Here's how the part is built. I have some questions about the finished solid (model axes, mm). Coordinates: 2 decimals unless noted, no trailing zeros. Write each loop counter-clockwise with the first axis right and the second up, starting at its lowest first coordinate (ties: lowest second). Pieces come first, ordered by that corner, then holes. Notation, with made-up numbers: M 82.5,-25.75 L 106.5,-25.75 A10 cw 106.5,-10.75 Z; hole C -30,16.5 d1. An arc over 180 degrees is marked long. Use a Markdown table: item, result.
```python
from build123d import *

# Parameters (mm, degrees)
SKETCH2_W                      = 53.34
SKETCH2_H                      = 17.780149528
BOSS_EXTRUDE1_DEPTH            = 1.524
F_2_CLEARANCE_HOLE1_AT_2_COUNT = 2
F_2_CLEARANCE_HOLE1_AT_2_PITCH = 13.038661485
F_2_CLEARANCE_HOLE1_AT_3_COUNT = 2
F_2_CLEARANCE_HOLE1_AT_3_PITCH = 50.333486658
F_2_CLEARANCE_HOLE1_AT_4_COUNT = 2
F_2_CLEARANCE_HOLE1_AT_4_PITCH = 48.615359567
FILLET1_R                      = 1.27
CUT_EXTRUDE1_REACH             = 30.154
SKETCH6_R                      = 6.35
FILLET2_R                      = 0.254


with BuildPart() as part:
    # Sketch2 → Boss-Extrude1 (new body)
    with BuildSketch(Plane.XY):
        Rectangle(SKETCH2_W, SKETCH2_H)
    extrude(amount=-BOSS_EXTRUDE1_DEPTH)

    # Sketch4 → #2 Clearance Hole1 (revolve, cut)
    with BuildSketch(Plane(origin=(-24.307679783, 6.519330742, 0), x_dir=(0, -1, 0), z_dir=(1, 0, 0))):
        Polygon((0, 0), (0, 1.524), (1.2192, 1.524), (1.2192, 0.635), (1.8542, 0), align=None)
    f_2_clearance_hole1 = revolve(axis=Axis((-24.307679783, 6.519330742, 6.35), (0, 0, -1)), mode=Mode.SUBTRACT)

    # #2 Clearance Hole1 at 2: #2 Clearance Hole1 ×2
    with Locations(*[(0, -i * F_2_CLEARANCE_HOLE1_AT_2_PITCH, 0) for i in range(1, F_2_CLEARANCE_HOLE1_AT_2_COUNT)]):
        add(f_2_clearance_hole1, mode=Mode.SUBTRACT)

    # #2 Clearance Hole1 at 3: #2 Clearance Hole1 ×2
    with Locations(*[Vector(0.9658651286657962, -0.25904546556040114, 0) * (i * F_2_CLEARANCE_HOLE1_AT_3_PITCH) for i in range(1, F_2_CLEARANCE_HOLE1_AT_3_COUNT)]):
        add(f_2_clearance_hole1, mode=Mode.SUBTRACT)

    # #2 Clearance Hole1 at 4: #2 Clearance Hole1 ×2
    with Locations(*[(i * F_2_CLEARANCE_HOLE1_AT_4_PITCH, 0, 0) for i in range(1, F_2_CLEARANCE_HOLE1_AT_4_COUNT)]):
        add(f_2_clearance_hole1, mode=Mode.SUBTRACT)

    # Fillet1
    fillet1_edges = [part.edges().sort_by_distance(p)[0] for p in [
        (-26.67, 8.890074764, -0.762),
        (26.67, 8.890074764, -0.762),
        (26.67, -8.890074764, -0.762),
        (-26.67, -8.890074764, -0.762),
    ]]
    fillet(fillet1_edges, radius=FILLET1_R)

    # Sketch6 → Cut-Extrude1 (cut, up to next)
    with BuildSketch(Plane.XY, mode=Mode.PRIVATE) as cut_extrude1_sk1:
        Circle(SKETCH6_R)
    cut_extrude1_tool1 = extrude(cut_extrude1_sk1.sketch, amount=-CUT_EXTRUDE1_REACH, mode=Mode.PRIVATE) & part.part
    # Sketch6 → Cut-Extrude1 (cut, up to next)
    with BuildSketch(Plane.XY, mode=Mode.PRIVATE) as cut_extrude1_sk2:
        with Locations((-17.78, 0)):
            Circle(SKETCH6_R)
    cut_extrude1_tool2 = extrude(cut_extrude1_sk2.sketch, amount=-CUT_EXTRUDE1_REACH, mode=Mode.PRIVATE) & part.part
    # Sketch6 → Cut-Extrude1 (cut, up to next)
    with BuildSketch(Plane.XY, mode=Mode.PRIVATE) as cut_extrude1_sk3:
        with Locations((17.779999999, -0.00017224)):
            Circle(SKETCH6_R)
    cut_extrude1_tool3 = extrude(cut_extrude1_sk3.sketch, amount=-CUT_EXTRUDE1_REACH, mode=Mode.PRIVATE) & part.part
    add(cut_extrude1_tool1.solids().sort_by_distance((0, 0, 0))[0], mode=Mode.SUBTRACT)
    add(cut_extrude1_tool2.solids().sort_by_distance((-17.78, 0, 0))[0], mode=Mode.SUBTRACT)
    add(cut_extrude1_tool3.solids().sort_by_distance((17.78, -0.000172, 0))[0], mode=Mode.SUBTRACT)

    # Fillet2
    fillet2_edges = [part.edges().sort_by_distance(p)[0] for p in [
        (0, 8.890074764, 0),
        (-26.67, 0, 0),
        (0, -8.890074764, 0),
        (26.67, 0, 0),
        (-26.298025612, -8.518100377, 0),
        (26.298025612, -8.518100377, 0),
        (26.298025612, 8.518100377, 0),
        (-26.298025612, 8.518100377, 0),
    ]]
    fillet(fillet2_edges, radius=FILLET2_R)


solid = part.part
```
1. Suppose I cut it at A-A on x = -17.78. Write out the boundary of the cut face in (y, z).
Answers follow:
| item | result |
|---|---|
| outline | M -8.89,-1.52 L -6.35,-1.52 L -6.35,0 L -8.64,0 A0.25 ccw -8.89,-0.25 Z; M 6.35,-1.52 L 8.89,-1.52 L 8.89,-0.25 A0.25 ccw 8.64,0 L 6.35,0 Z |
2. Suppose I cut it at C-C on y = -7. State how many separate pieces and enclosed holes the cut face has, and give its area (3 significant figures).
Answers follow:
| item | result |
|---|---|
| separate pieces | 3 |
| enclosed holes | 0 |
| area | 73.6 mm2 |
3. Will this pin go through, and if not, where does the flat tip stop? pin 1 Ø3 at (x, y) = (24.31, -6.52) entering from +Z.
Answers follow:
| item | result |
|---|---|
| pin 1 | stops at z = -0.35 |
4. I need wall thicknesses on probe 1 along Y at (x, z) = (17.5, -1.05); probe 2 along X at (y, z) = (5, -0.5); probe 3 along X at (y, z) = (-4, -1.2). Which ranges of each line are inside material? Lowest first, please.
Answers follow:
| item | result |
|---|---|
| probe 1 | y = -8.89 to -6.34, 6.34 to 8.89 |
| probe 2 | x = -26.67 to -21.69, -13.87 to -3.91, 3.91 to 13.87, 21.69 to 26.67 |
| probe 3 | x = -26.67 to -22.71, -12.85 to -4.93, 4.93 to 12.85, 22.71 to 26.67 |
5. We'd pull the mould along X, two halves only. Please class faces 1 (the face through (-24.124, 0.279, -0.751)), 2 (the face through (-6.2, 2, 0)), 3 (the face through (26.67, 0, -1)): +X half, -X half, draft (parallel to the pull), parting line (faces both ways), or undercut.
Answers follow:
| item | result |
|---|---|
| face 1 | undercut |
| face 2 | draft |
| face 3 | +X half |
6. Suppose I cut it at D-D on x = -2. Write out the boundary of the cut face in (y, z), and give its area (3 significant figures).
Answers follow:
| item | result |
|---|---|
| outline | M -8.89,-1.52 L -6.03,-1.52 L -6.03,0 L -8.64,0 A0.25 ccw -8.89,-0.25 Z; M 6.03,-1.52 L 8.89,-1.52 L 8.89,-0.25 A0.25 ccw 8.64,0 L 6.03,0 Z |
| area | 8.70 mm2 |
7. Suppose I cut it at B-B on z = -1. Write out the boundary of the cut face in (x, y).
Answers follow:
| item | result |
|---|---|
| outline | M -26.67,-7.62 A1.27 ccw -25.4,-8.89 L 25.4,-8.89 A1.27 ccw 26.67,-7.62 L 26.67,7.62 A1.27 ccw 25.4,8.89 L -25.4,8.89 A1.27 ccw -26.67,7.62 Z; hole C -24.31,-6.52 d2.44; hole C -24.31,6.52 d2.44; hole C -17.78,0 d12.7; hole C 0,0 d12.7; hole C 17.78,0 d12.7; hole C 24.31,-6.52 d2.44; hole C 24.31,6.52 d2.44 |
